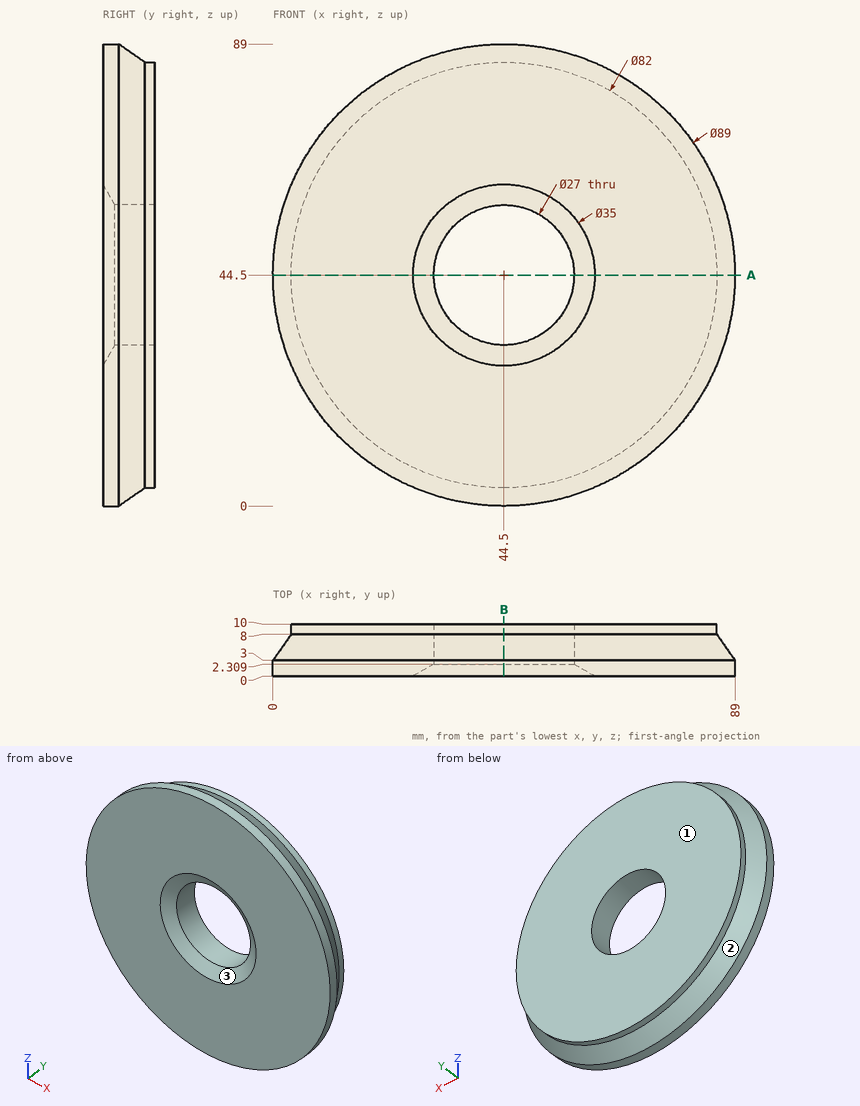
Geometry: see drawing. Coordinates: mm, zero at the bounding-box minimum. Coordinates: 2 decimals unless noted, no trailing zeros. Write each loop counter-clockwise with the first axis right and the second up, starting at its lowest first coordinate (ties: lowest second). Pieces come first, ordered by that corner, then holes.
1) Section A-A on z = 44.5. Output: boundary loops of the cut face in (x, y), and give its area (3 significant figures).
2) Section B-B on x = 44.5. Output: boundary loops of the cut face in (y, z), and give its area (3 significant figures).
3) Mould query, pull axis X, two halves, no side actions, for the marked faces 1, 2 and 3. Classes: pulls with the +X half, pulls with the -X half, needs draft (parallel to the pull), parting line crosses it, or undercut.
4) Pin query (flat end, axial travel): pin 1 Ø2 at (x, z) = (48, 67) entering from -Y; pin 2 Ø5 at (y, z) = (3, 31) entering from +X; pin 3 Ø6 at (x, y) = (31.5, 4.5) entering from +Z; pin 4 Ø1.5 at (y, z) = (1, 64.5) entering from +X. Return the tip coordinate at first contact, or that it passes through.
5) Material intervals for line 1 along X through (y, z) = (7.5, 44.5); line 2 along X through (y, z) = (8.25, 35) (1 decimal); line 3 along Z through (x, y) = (52, 4.5) (1 decimal), sorted ascending.
Check result:
1. outline: (0, 0) - (27, 0) - (31, 2.31) - (31, 10) - (3.5, 10) - (3.5, 8) - (0, 3) - close; (58, 2.31) - (62, 0) - (89, 0) - (89, 3) - (85.5, 8) - (85.5, 10) - (58, 10) - close
1. area: 579 mm2
2. outline: (0, 0) - (3, 0) - (8, 3.5) - (10, 3.5) - (10, 31) - (2.31, 31) - (0, 27) - close; (0, 62) - (2.31, 58) - (10, 58) - (10, 85.5) - (8, 85.5) - (3, 89) - (0, 89) - close
2. area: 579 mm2
3. face 1: needs draft
3. face 2: parting line crosses it
3. face 3: undercut
4. pin 1: stops at y = 0
4. pin 2: stops at x = 87.62
4. pin 3: stops at z = 87.77
4. pin 4: stops at x = 84.62
5. line 1: x = 3.15 to 31, 58 to 85.85
5. line 2: x = 4.6 to 34.9, 54.1 to 84.4
5. line 3: z = 1.7 to 33.3, 55.7 to 87.3
